For this review, take the finished solid that the model builds, in its own axes (mm). A direction names the side the tool comes from. Coordinates: 2 decimals unless noted, no trailing zeros. Loops run counter-clockwise (first coordinate to the right, second up) from the corner with the lowest first, then second, coordinate; pieces in that order, holes last. Notation, with made-up numbers: M 23.25,1 L 56.25,1 A17 cw 56.25,21 Z; hole C 9,36.5 d3. An arc over 180 degrees is marked long. Answer as a JSON object with one key per item and string values. Group by question number.
Item 1: Add section D-D (z = 7). State the section outline as (x, y) points, then the cut area to 3 significant figures.
Item 2: Add section C-C (y = -37.5). State the section outline as (x, z) points, then the cut area to 3 significant figures.
Item 3: Mouldability with a two-part tool opening along X and no side actions: class faces 3 (the face through (13.48, -17.26, 3.94)), 4 (the face through (0, -19, 8)), 5 (the face through (-3.669, -28.803, 1.014)) as +X half, -X half, draft (parallel to the pull), parting line (faces both ways), or undercut.
Item 4: Insertion check: pin 1 (2 mm diameter, centred on x = 1, z = 2, fed in from +Y); pin 2 (1 mm diameter, centred on x = 2, z = 1.5, fed in from -Y); pin 3 (7.5 mm diameter, centred on x = -5, y = -31.5, fed in from +Z); pin 4 (2 mm diameter, centred on y = -39.5, z = 4.5, fed in from +X). Each pin has a flat end and moves straight along its axis. Give the tip position at first contact, or say it passes through.
Item 5: Add section A-A (x = 0). State the section outline as (y, z) points.
Item 6: Tool access review of faces 1 (the face through (6.72, -24.46, 5.04)), 2 (the face through (-13.52, -17.74, 3.94)): name each direction out of +Z, -Z, +X, -X, +Y, -Y from which nothing blocks a thin tool from reaching the whole face with its end or side.
Item 7: Wall thickness on L1, parallel to Y at x = 0, z = 0.85; L2, parallel to Y at x = 0, z = 6.3; L3, parallel to Y at x = -4.5, z = 0.85: over which ranges is each line inside the solid? List them lowest first. Write a range as from..to.
Item 8: Add section B-B (x = 9). State the section outline as (y, z) points, then the cut area to 3 significant figures.
from build123d import *

# Parameters (mm, degrees)
BOSS_EXTRU_1_DEPTH      = 8
ESQUISSE2_R             = 6.5
ENL_V_MAT_EXTRU_1_DEPTH = 10
ESQUISSE3_R             = 1.8
ENL_V_MAT_EXTRU_2_DEPTH = 10
ESQUISSE5_R             = 12.5
ENL_V_MAT_EXTRU_5_DEPTH = 6
ESQUISSE19_R            = 8.1
ENL_V_MAT_EXTRU_6_DEPTH = 10
BOSS_EXTRU_2_START      = -3
ESQUISSE22_R            = 8.1
ESQUISSE22_R_2          = 5
BOSS_EXTRU_2_DEPTH      = 3


with BuildPart() as part:
    # Esquisse1 → Boss.-Extru.1 (new body)
    with BuildSketch(Plane.XY):
        with BuildLine():
            Line((12, 0), (15, -35))
            ThreePointArc((15, -35), (0, -50), (-15, -35))
            Line((-15, -35), (-12, 0))
            ThreePointArc((-12, 0), (0, 12), (12, 0))
        make_face()
    extrude(amount=BOSS_EXTRU_1_DEPTH)

    # Esquisse2 → Enlèv. mat.-Extru.1 (cut)
    with BuildSketch(Plane.XY.offset(8)):
        with Locations((0, -35)):
            Circle(ESQUISSE2_R)
    extrude(amount=-ENL_V_MAT_EXTRU_1_DEPTH, mode=Mode.SUBTRACT)

    # Esquisse3 → Enlèv. mat.-Extru.2 (cut)
    with BuildSketch(Plane.XY.offset(8)):
        with Locations((9, -35)):
            Circle(ESQUISSE3_R)
        with Locations((-4.5, -27.205771366)):
            Circle(ESQUISSE3_R)
        with Locations((-4.5, -42.794228634)):
            Circle(ESQUISSE3_R)
    extrude(amount=-ENL_V_MAT_EXTRU_2_DEPTH, mode=Mode.SUBTRACT)

    # Esquisse5 → Enlèv. mat.-Extru.5 (cut)
    with BuildSketch(Plane.XY.offset(8)):
        with Locations((0, -35)):
            Circle(ESQUISSE5_R)
    extrude(amount=-ENL_V_MAT_EXTRU_5_DEPTH, mode=Mode.SUBTRACT)

    # Esquisse19 → Enlèv. mat.-Extru.6 (cut)
    with BuildSketch(Plane.XY.offset(8)):
        Circle(ESQUISSE19_R)
    extrude(amount=-ENL_V_MAT_EXTRU_6_DEPTH, mode=Mode.SUBTRACT)

    # Esquisse22 → Boss.-Extru.2 (add)
    with BuildSketch(Plane(origin=(0, 0, 0), x_dir=(-1, 0, 0), z_dir=(0, 0, -1)).offset(BOSS_EXTRU_2_START)):
        with Locations(Location((0, 0, 0), (0, 0, 180))):
            Circle(ESQUISSE22_R)
        Circle(ESQUISSE22_R_2, mode=Mode.SUBTRACT)
    extrude(amount=BOSS_EXTRU_2_DEPTH)


solid = part.part
From the geometry:
{
 "1": {"outline": "M -15,-35 A15 ccw 15,-35 L 12,0 A12 ccw -12,0 Z; hole C 0,-35 d25; hole C 0,0 d16.2", "area": "828 mm²"},
 "2": {"outline": "M -14.79,0 L -6,0 L -6,2 L -12.25,2 L -12.25,8 L -14.79,8 Z; M 6,0 L 14.79,0 L 14.79,8 L 12.25,8 L 12.25,2 L 6,2 Z", "area": "65.7 mm²"},
 "3": {"face 3": "+X half", "face 4": "draft", "face 5": "undercut"},
 "4": {"pin 1": "stops at y = 12", "pin 2": "stops at y = -49.92", "pin 3": "stops at z = 2", "pin 4": "stops at x = 14.59"},
 "5": {"outline": "M -50,0 L -41.5,0 L -41.5,2 L -47.5,2 L -47.5,8 L -50,8 Z; M -28.5,0 L -5,0 L -5,3 L -8.1,3 L -8.1,8 L -22.5,8 L -22.5,2 L -28.5,2 Z; M 5,0 L 12,0 L 12,8 L 8.1,8 L 8.1,3 L 5,3 Z"},
 "6": {"face 1": "+Z", "face 2": "+Z, -Z, -X, +Y"},
 "7": {"L1": "y = -50..-41.5, -28.5..-5, 5..12", "L2": "y = -50..-47.5, -22.5..-8.1, 8.1..12", "L3": "y = -49.31..-44.59, -40.99..-39.69, -30.31..-29.01, -25.41..-2.18, 2.18..11.12"},
 "8": {"outline": "M -47,0 L -36.8,0 L -36.8,2 L -43.67,2 L -43.67,8 L -47,8 Z; M -33.2,0 L 7.94,0 L 7.94,8 L -26.33,8 L -26.33,2 L -33.2,2 Z", "area": "328 mm²"}
}
